Part print with two shaded views. Sizes in mm from the minimum x, y, z corner. A direction names the side the tool comes from. Give positions to 0.01 mm unless a question says otherwise; leave off trailing zeros. Write each loop counter-clockwise with the first axis right and the second up, starting at its lowest first coordinate (ties: lowest second). Pieces come first, ordered by that corner, then holes. Notation, with made-up numbers: (-25, 85) -> (-9, 85) arc R29 ccw to (-9, 120) -> close; hole circle Ø3 at (4, 57.5). An arc over 180 degrees is marked (long way). Answer as a JSON object with one key per item and string values.
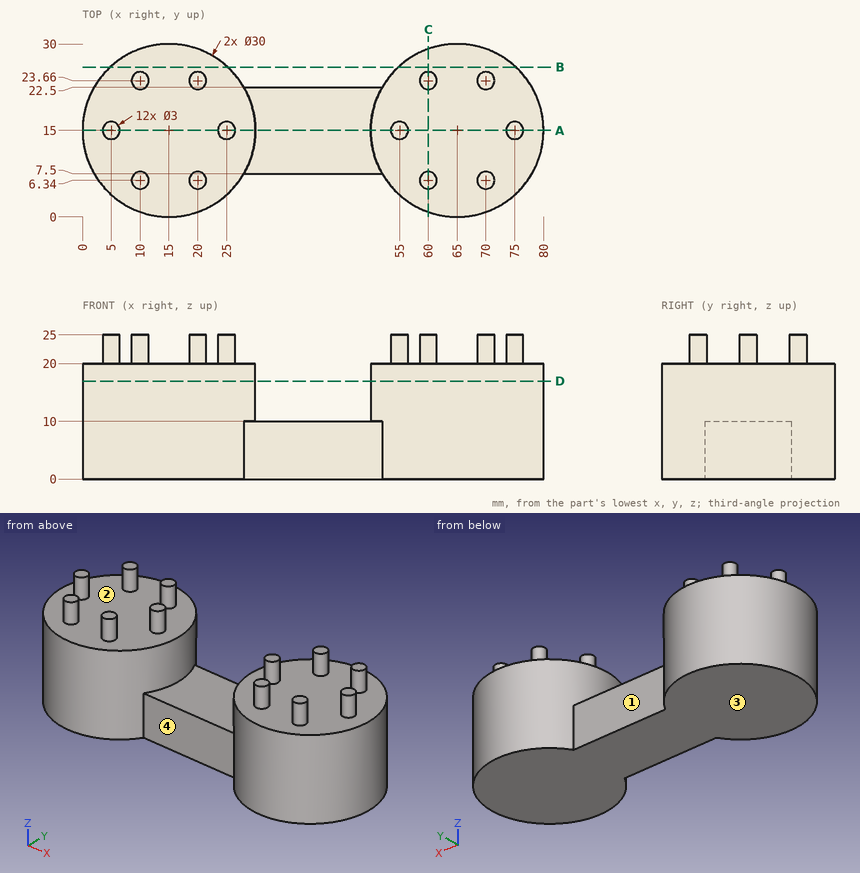
1) Slice it at A-A (y = 15). List the corners of the cut face in (x, z), then the cut area to 3 significant figures.
Model answer:
{"outline": "(0, 0) -> (80, 0) -> (80, 20) -> (76.5, 20) -> (76.5, 25) -> (73.5, 25) -> (73.5, 20) -> (56.5, 20) -> (56.5, 25) -> (53.5, 25) -> (53.5, 20) -> (50, 20) -> (50, 10) -> (30, 10) -> (30, 20) -> (26.5, 20) -> (26.5, 25) -> (23.5, 25) -> (23.5, 20) -> (6.5, 20) -> (6.5, 25) -> (3.5, 25) -> (3.5, 20) -> (0, 20) -> close", "area": "1,460 mm2"}
2) Pin check, flat tips, straight feed: pin 1 (3 mm diameter, centred on x = 15.5, y = 13, fed in from -Z); pin 2 (5 mm diameter, centred on x = 46, z = 6, fed in from +Y); pin 3 (1.5 mm diameter, centred on y = 9.5, z = 9.5, fed in from +X); pin 4 (12 mm diameter, centred on x = 38.5, y = 17, fed in from +Z). Stop position of each tip, or through.
Model answer:
{"pin 1": "stops at z = 0", "pin 2": "stops at y = 22.5", "pin 3": "stops at x = 79.23", "pin 4": "stops at z = 10"}
3) Slice it at C-C (x = 60). List the corners of the cut face in (y, z).
Model answer:
{"outline": "(0.86, 0) -> (29.14, 0) -> (29.14, 20) -> (25.16, 20) -> (25.16, 25) -> (22.16, 25) -> (22.16, 20) -> (7.84, 20) -> (7.84, 25) -> (4.84, 25) -> (4.84, 20) -> (0.86, 20) -> close"}
4) Slice it at B-B (y = 26). List the corners of the cut face in (x, z), then the cut area to 3 significant figures.
Model answer:
{"outline": "(4.8, 0) -> (25.2, 0) -> (25.2, 20) -> (4.8, 20) -> close; (54.8, 0) -> (75.2, 0) -> (75.2, 20) -> (54.8, 20) -> close", "area": "816 mm2"}
5) Wall check: probe 1 along X at (y, z) = (6, 20.25); probe 2 along Z at (x, y) = (56, 19.75); probe 3 along Y at (x, z) = (52, 11) (1 decimal). Give the ranges that are in metal, low to high.
Model answer:
{"probe 1": "x = 8.54 to 11.46, 18.54 to 21.46, 58.54 to 61.46, 68.54 to 71.46", "probe 2": "z = 0 to 20", "probe 3": "y = 7.5 to 22.5"}
6) 3-axis set-ups, long thin cutter, end or side, ignore diameter. For the marked faces 1 and 2: which of +Z, -Z, +X, -X, +Y, -Y reach the whole face in a straight line?
Model answer:
{"face 1": "+Z, -Z, +Y", "face 2": "+Z"}
7) Slice it at D-D (z = 17). List the corners of the cut face in (x, y), then the cut area to 3 significant figures.
Model answer:
{"outline": "circle Ø30 at (15, 15); circle Ø30 at (65, 15)", "area": "1,410 mm2"}
8) Mould opens along X. For the marked faces 3 and 4 say: released by +X, released by -X, zero draft, split by the parting line, or undercut.
Model answer:
{"face 3": "zero draft", "face 4": "undercut"}
